from build123d import *

# Parameters (mm, degrees)
F0_W     = 50
F0_H     = 50
F1_DEPTH = 5
F3_D     = 5
F5_D     = 5


with BuildPart() as f1:
    # F0 (on Top) → F1 (new body)
    with BuildSketch(Plane.XY):
        Rectangle(F0_W, F0_H)
    extrude(amount=F1_DEPTH)

    # F3 (through all)
    with Locations(Plane.XY.offset(5)):
        with Locations((-10.019323, 10.674792)):
            Hole(F3_D / 2)

    # F5 (through all)
    with Locations(Plane.XY.offset(5)):
        with Locations((-15, 15), (15, 15), (15, -15), (-15, -15)):
            Hole(F5_D / 2)


solid = f1.part
Design review of the part built by this model. Coordinates are the model's own, in mm. Round coordinates to 2 decimals unless told otherwise and drop trailing zeros. Loops run counter-clockwise (first coordinate to the right, second up) from the corner with the lowest first, then second, coordinate; pieces in that order, holes last. Notation, with made-up numbers: (42, -38) - (47, -38) arc R15 cw to (47, -10) - close; hole circle Ø10 at (84.25, -24). An arc over 180 degrees is marked (long way). One line per item, written item: value. Start each with the question number.
1) Draft analysis for pull direction X (two halves, no side actions). For faces 1 (the cylindrical face through (-12.5, -14.9, 2.5)), 2 (the flat face through (0, 25, 2)), 3 (the flat face through (-25, 0, 2)), state which applies: +X half, -X half, draft (parallel to the pull), parting line (faces both ways), or undercut.
2) To check wall thickness, follow L1, parallel to Y at x = 15, z = 1.6; L2, parallel to Y at x = -14.5, z = 1.1; L3, parallel to X at y = 16.5, z = 4.45. State the ranges of each line that lie inside material, in increasing order. Write a range as from..to.
3) Consider section A-A on y = -15. Give the boundary of the cut face in (x, z), then the cut area to 3 significant figures.
4) Consider section C-C on z = 1.7. Give the boundary of the cut face in (x, y), then the cut area to 3 significant figures.
Reported:
1. face 1: undercut
1. face 2: draft
1. face 3: -X half
2. L1: y = -25..-17.5, -12.5..12.5, 17.5..25
2. L2: y = -25..-17.45, -12.55..12.55, 17.45..25
2. L3: x = -25..-17, -13..13, 17..25
3. outline: (-25, 0) - (-17.5, 0) - (-17.5, 5) - (-25, 5) - close; (-12.5, 0) - (12.5, 0) - (12.5, 5) - (-12.5, 5) - close; (17.5, 0) - (25, 0) - (25, 5) - (17.5, 5) - close
3. area: 200 mm^2
4. outline: (-25, -25) - (25, -25) - (25, 25) - (-25, 25) - close; hole circle Ø5 at (-15, -15); hole circle Ø5 at (-15, 15); hole circle Ø5 at (-10.02, 10.67); hole circle Ø5 at (15, -15); hole circle Ø5 at (15, 15)
4. area: 2,400 mm^2
